Can you work these out from the model? Positions are in its coordinate system, mm. A direction names the side the tool comes from. Coordinates: 2 decimals unless noted, no trailing zeros. Write each loop counter-clockwise with the first axis right and the second up, starting at its lowest first coordinate (ties: lowest second). Pieces come first, ordered by that corner, then holes. Notation, with made-up numbers: (34, 67.5) - (87, 67.5) arc R23 ccw to (87, 95.5) - close; hole circle Ø2 at (23, -39.75). An arc over 180 degrees is marked (long way). Use one line per item in the form item = value. Start each with the question number.
(1) If we section it at A-A on y = -25.4: Please give me the cut outline in (x, z), then the cut area to 3 significant figures.
(2) On a 3-axis mill with a long thin cutter (end or side, diameter ignored), from which of +Z, -Z, +X, -X, +Y, -Y can I reach the whole of each face in a straight line? I mean faces 1 (the face through (0, -91, 29)), 2 (the face through (6.35, -75, 36)), 3 (the face through (2, -152.4, 55)), 4 (the face through (61.689, -75.133, 53.687)), 5 (the face through (32, -171, 52.07)). Say none if no direction works.
(3) For pin 1 Ø5 at (x, z) = (53.5, 25) entering from -Y; pin 2 Ø1.9 at (x, z) = (3, 55) entering from +Y; pin 3 Ø6 at (x, z) = (17.5, 17) entering from -Y; pin 4 Ø0.8 at (y, z) = (-69, 56.5) entering from +X, each with a flat end and sliding along its axis, tell me the tip position at first contact or that it passes through.
(4) If we section it at D-D on x = 33.5: Please give me the cut outline in (y, z), then the cut area to 3 significant figures.
(5) If we section it at C-C on y = -95.25: Please give me the cut outline in (x, z).
(6) If we section it at B-B on z = 9.5: Please give me the cut outline in (x, y).
(7) Thinking about a two-plate mould opening in X: for faces 6 (the face through (31, -152.4, 26)), 7 (the face through (7.64, -202.31, 21.82)), 8 (the face through (61, -152.4, 55)), which applies, pulls with the +X half, pulls with the -X half, needs draft (parallel to the pull), parting line crosses it, or undercut?
(8) If I drill on probe 1 along X at (y, z) = (-89.5, 49); probe 2 along Y at (x, z) = (32, 8); probe 3 along X at (y, z) = (-172.5, 21), over which ranges is the centre line in solid material (lowest first)? Write a range as from..to.
```python
from build123d import *

# Parameters (mm, degrees)
F1_DEPTH     = 152.4
F2_W         = 50.8
F2_H         = 50.8
F3_DEPTH     = 57.15
F4_R         = 25.4
F5_T         = 5.08
F5_T3_DEPTH  = 11.7136995755
F5_T5_DEPTH  = 162.56
F5_T7_DEPTH  = 60.96
F5_T9_DEPTH  = 60.96
F5_T12_ANGLE = 90.000000001
F5_T14_ANGLE = 90.000000001
F6_R         = 6.35
F7_DEPTH     = 63.501
F8_R         = 6.35
F9_DEPTH     = 57.151


# Not quite as in the source:
# - a shell that OpenCascade refuses in one call is made with other operations: the cavity is built on its own and cut out


with BuildPart() as f1:
    # F0 (on Front) → F1 (new body)
    with BuildSketch(Plane.XZ):
        with BuildLine():
            Line((0, 49.2463004245), (0, 0))
            Line((0, 0), (6.35, 0))
            Line((6.35, 0), (6.35, 50.8))
            Line((6.35, 50.8), (57.15, 50.8))
            Line((57.15, 50.8), (57.15, 0))
            Line((57.15, 0), (63.5, 0))
            Line((63.5, 0), (63.5, 49.2463004245))
            ThreePointArc((63.5, 49.2463004245), (61.6401280605, 53.736428485), (57.15, 55.5963004245))
            Line((57.15, 55.5963004245), (57.15, 57.15))
            Line((57.15, 57.15), (6.35, 57.15))
            Line((6.35, 57.15), (6.35, 55.5963004245))
            ThreePointArc((6.35, 55.5963004245), (1.8598719395, 53.736428485), (0, 49.2463004245))
        make_face()
    extrude(amount=F1_DEPTH)

    # F2 (on face) → F3 (join)
    with BuildSketch(Plane.XZ.offset(152.4)):
        with BuildLine():
            Line((0, 49.2463004245), (0, 0))
            Line((0, 0), (6.35, 0))
            Line((6.35, 0), (6.35, 50.8))
            Line((6.35, 50.8), (57.15, 50.8))
            Line((57.15, 50.8), (57.15, 0))
            Line((57.15, 0), (63.5, 0))
            Line((63.5, 0), (63.5, 49.2463004245))
            ThreePointArc((63.5, 49.2463004245), (61.6401280605, 53.736428485), (57.15, 55.5963004245))
            Line((57.15, 55.5963004245), (57.15, 57.15))
            Line((57.15, 57.15), (6.35, 57.15))
            Line((6.35, 57.15), (6.35, 55.5963004245))
            ThreePointArc((6.35, 55.5963004245), (1.8598719395, 53.736428485), (0, 49.2463004245))
        make_face()
        with BuildLine():
            Line((0, 57.15), (0, 49.2463004245))
            ThreePointArc((0, 49.2463004245), (1.8598719395, 53.736428485), (6.35, 55.5963004245))
            Line((6.35, 55.5963004245), (6.35, 57.15))
            Line((6.35, 57.15), (0, 57.15))
        make_face()
        with BuildLine():
            ThreePointArc((57.15, 55.5963004245), (61.6401280605, 53.736428485), (63.5, 49.2463004245))
            Line((63.5, 49.2463004245), (63.5, 57.15))
            Line((63.5, 57.15), (57.15, 57.15))
            Line((57.15, 57.15), (57.15, 55.5963004245))
        make_face()
        with Locations((31.75, 25.4)):
            Rectangle(F2_W, F2_H)
    extrude(amount=F3_DEPTH)

    # F4
    f4_edges = [f1.edges().sort_by_distance(p)[0] for p in [
        (31.75, -209.55, 57.15),
        (0, -209.55, 28.575),
        (63.5, -209.55, 28.575),
    ]]
    fillet(f4_edges, radius=F4_R)

    # F5: shell of thickness 5.08, made by hand


with BuildPart() as f5_core1:
    # F5_t2: copy of F1
    add(f1.part)

    # the walls: a layer under each face that stays
    f5_faces = [f5_core1.faces().sort_by_distance(p)[0] for p in [
        (0, -92.075, 28.575),
        (31.75, -92.075, 57.15),
        (7.4394877579, -202.1105122421, 28.575),
        (1.0583333333, -152.4, 53.1981502122),
        (1.8598719395, -76.2, 53.736428485),
        (4.5357142857, 0, 4.0821428571),
        (63.5, -92.075, 28.575),
        (31.75, -202.1105122421, 49.7105122421),
        (58.2083333333, -152.4, 55.8327167374),
        (57.15, -76.2, 56.3731502122),
        (6.35, -76.2, 56.3731502122),
        (31.75, -209.55, 15.875),
        (6.35, -76.2, 25.4),
        (56.0605122421, -202.1105122421, 28.575),
        (31.75, -152.4, 25.4),
        (57.15, -76.2, 25.4),
        (31.75, -76.2, 50.8),
        (61.6401280605, -76.2, 53.736428485),
    ]]
    thicken(f5_faces, amount=-F5_T, mode=Mode.SUBTRACT)

    # F5_s4 → F5_t3 (cut)
    with BuildSketch(Plane.XY.offset(50.5163004245)):
        Polygon((6.2992, -152.3492), (6.35, -157.48), (11.43, -157.48), (11.43, -152.4), align=None)
        Polygon((57.2008, -152.3492), (57.15, -157.48), (52.07, -157.48), (52.07, -152.4), align=None)
    extrude(amount=F5_T3_DEPTH, mode=Mode.SUBTRACT)

    # F5_s6 → F5_t5 (cut)
    with BuildSketch(Plane.XZ.offset(-5.08)):
        Polygon((6.2992, 55.6471004245), (6.35, 50.5163004245), (11.43, 50.5163004245), (11.43, 55.5963004245), align=None)
        Polygon((57.2008, 55.6471004245), (52.07, 55.5963004245), (52.07, 50.5163004245), (57.15, 50.5163004245), align=None)
        Polygon((6.4008, 50.7492), (1.27, 50.8), (1.27, 55.88), (6.35, 55.88), align=None)
        Polygon((57.0992, 50.7492), (62.23, 50.8), (62.23, 55.88), (57.15, 55.88), align=None)
    extrude(amount=F5_T5_DEPTH, mode=Mode.SUBTRACT)

    # F5_s8 → F5_t7 (cut)
    with BuildSketch(Plane.XY.offset(-5.08)):
        Polygon((6.4008, -152.3492), (1.27, -152.4), (1.27, -157.48), (6.35, -157.48), align=None)
        Polygon((57.0992, -152.3492), (57.15, -157.48), (62.23, -157.48), (62.23, -152.4), align=None)
    extrude(amount=F5_T7_DEPTH, mode=Mode.SUBTRACT)

    # F5_s10 → F5_t9 (cut)
    with BuildSketch(Plane.YZ.offset(1.27)):
        Polygon((-152.3492, 50.7492), (-157.48, 50.8), (-157.48, 55.88), (-152.4, 55.88), align=None)
    extrude(amount=F5_T9_DEPTH, mode=Mode.SUBTRACT)

    # F5_s11 → F5_t12 (revolve, cut)
    with BuildSketch(Plane.YZ.offset(6.35)):
        Polygon((-152.3492, 55.6471004245), (-157.48, 55.5963004245), (-157.48, 50.5163004245), (-152.4, 50.5163004245), align=None)
    revolve(axis=Axis((6.35, -152.4, 49.2463004245), (0, -1, 0)), revolution_arc=F5_T12_ANGLE, mode=Mode.SUBTRACT)

    # F5_s13 → F5_t14 (revolve, cut)
    with BuildSketch(Plane.XY.offset(49.2463004245)):
        Polygon((63.5508, -152.3492), (63.5, -157.48), (58.42, -157.48), (58.42, -152.4), align=None)
    revolve(axis=Axis((57.15, -152.4, 49.2463004245), (0, -1, 0)), revolution_arc=F5_T14_ANGLE, mode=Mode.SUBTRACT)


with BuildPart() as f1_1:
    add(f1.part)

    # what is left inside the walls is the cavity
    f5_cavity = [f5_core1.part.solids().sort_by_distance(p)[0] for p in [
        (31.75, -157.5308, 34.713333),
    ]]
    add(f5_cavity, mode=Mode.SUBTRACT)

    # F6 (on face) → F7 (cut, through all)
    with BuildSketch(Plane(origin=(0, 0, 0), x_dir=(0, -1, 0), z_dir=(-1, 0, 0))):
        with Locations((25.4, 24.6231502122)):
            Circle(F6_R)
        with Locations((76.2, 24.6231502122)):
            Circle(F6_R)
    extrude(amount=-F7_DEPTH, mode=Mode.SUBTRACT)

    # F8 (on face) → F9 (cut, through all)
    with BuildSketch(Plane.XY.offset(57.15)):
        with Locations((31.75, -44.45)):
            Circle(F8_R)
        with Locations((31.75, -95.25)):
            Circle(F8_R)
    extrude(amount=-F9_DEPTH, mode=Mode.SUBTRACT)


solid = f1_1.part
```
Reported:
q1.outline = (0, 0) - (6.35, 0) - (6.35, 18.27) - (0, 18.27) - close; (0, 30.97) - (6.35, 30.97) - (6.35, 50.8) - (57.15, 50.8) - (57.15, 30.97) - (63.5, 30.97) - (63.5, 49.25) arc R6.35 ccw to (57.15, 55.6) - (57.15, 57.15) - (6.35, 57.15) - (6.35, 55.6) arc R6.35 ccw to (0, 49.25) - close; (57.15, 0) - (63.5, 0) - (63.5, 18.27) - (57.15, 18.27) - close
q1.area = 850 mm2
q2.face_1 = +Z, -Z, -X, +Y, -Y
q2.face_2 = -Z, +Y
q2.face_3 = +Z, -X, +Y
q2.face_4 = +Z, +X, +Y
q2.face_5 = -Z
q3.pin_1 = -206.03
q3.pin_2 = 0
q3.pin_3 = -209.07
q3.pin_4 = 57.15
q4.outline = (-209.55, 0) - (-204.47, 0) - (-204.47, 31.75) arc R20.32 cw to (-184.15, 52.07) - (-157.48, 52.07) - (-157.48, 0) - (-152.4, 0) - (-152.4, 50.8) - (-101.35, 50.8) - (-101.35, 57.15) - (-184.15, 57.15) arc R25.4 ccw to (-209.55, 31.75) - close; (-89.15, 50.8) - (-50.55, 50.8) - (-50.55, 57.15) - (-89.15, 57.15) - close; (-38.35, 50.8) - (0, 50.8) - (0, 57.15) - (-38.35, 57.15) - close
q4.area = 1,580 mm2
q5.outline = (0, 0) - (6.35, 0) - (6.35, 50.8) - (25.4, 50.8) - (25.4, 57.15) - (6.35, 57.15) - (6.35, 55.6) arc R6.35 ccw to (0, 49.25) - close; (38.1, 50.8) - (57.15, 50.8) - (57.15, 0) - (63.5, 0) - (63.5, 49.25) arc R6.35 ccw to (57.15, 55.6) - (57.15, 57.15) - (38.1, 57.15) - close
q6.outline = (0, -184.15) arc R25.4 ccw to (25.4, -209.55) - (38.1, -209.55) arc R25.4 ccw to (63.5, -184.15) - (63.5, 0) - (57.15, 0) - (57.15, -152.4) - (6.35, -152.4) - (6.35, 0) - (0, 0) - close; hole (5.08, -184.15) arc R20.32 ccw to (25.4, -204.47) - (38.1, -204.47) arc R20.32 ccw to (58.42, -184.15) - (58.42, -157.48) - (5.08, -157.48) - close
q7.face_6 = undercut
q7.face_7 = pulls with the -X half
q7.face_8 = needs draft
q8.probe_1 = 0..6.35, 57.15..63.5
q8.probe_2 = -209.55..-204.47, -157.48..-152.4
q8.probe_3 = 0..5.08, 58.42..63.5
